Here's how the part is built. I have some questions about the finished solid (model axes, mm). Face numbers are marked on the shaded views. Round coordinates to 2 decimals unless told otherwise and drop trailing zeros. Write each loop counter-clockwise with the first axis right and the second up, starting at its lowest first coordinate (ties: lowest second). Pieces come first, ordered by that corner, then holes. Notation, with made-up numbers: (-13, -19) - (42, -19) arc R20 ccw to (42, 18) - close; hole circle Ø1 at (61.5, 25.5). An arc over 180 degrees is marked (long way). One line per item, written item: value. Start each with the question number.
Item 1: If I drill on line 1 (Z direction, x = -4, y = 10); line 2 (X direction, y = -0.5, z = 6); line 3 (Y direction, x = -14, z = 7.5), over which ranges is the centre line in solid material (lowest first)?
Item 2: Imagine slicing it at B-B, the plane x = 0. Please give me the cut outline in (y, z), then the cut area to 3 significant figures.
Item 3: For P1, Ø10, axis at x = 0.5, y = 0.5, coming from the +Z side, with a flat end and sliding along its axis, tell me the tip position at first contact or that it passes through.
Item 4: Thinking about a two-plate mould opening in X: for the marked faces 1, 2, 3 and 4, which applies, released by +X, released by -X, zero draft, split by the parting line, or undercut?
Item 5: Imagine slicing it at A-A, the plane z = 10.25. Please give me the cut outline in (x, y).
```python
from build123d import *

# Parameters (mm, degrees)
F0_W     = 74
F0_H     = 37
F1_DEPTH = 16
F2_T     = -1.5
F3_W     = 74
F3_H     = 37
F3_W_2   = 72
F3_H_2   = 35
F4_DEPTH = 2
F5_R     = 2


with BuildPart() as f1:
    # F0 (on Top) → F1 (new body)
    with BuildSketch(Plane.XY):
        Rectangle(F0_W, F0_H)
    extrude(amount=F1_DEPTH)

    # F2 (hollow: no face is removed)
    offset(amount=F2_T, mode=Mode.SUBTRACT)

    # F3 (on face) → F4 (join)
    with BuildSketch(Plane.XY.offset(16)):
        Rectangle(F3_W, F3_H)
        Rectangle(F3_W_2, F3_H_2, mode=Mode.SUBTRACT)
    extrude(amount=F4_DEPTH)

    # F5
    f5_edges = [f1.edges().sort_by_distance(p)[0] for p in [
        (-37, -18.5, 9),
        (36, 17.5, 17),
        (-36, 17.5, 17),
        (-36, -17.5, 17),
        (36, -17.5, 17),
        (37, -18.5, 9),
        (-37, 18.5, 9),
        (37, 18.5, 9),
    ]]
    fillet(f5_edges, radius=F5_R)


solid = f1.part
```
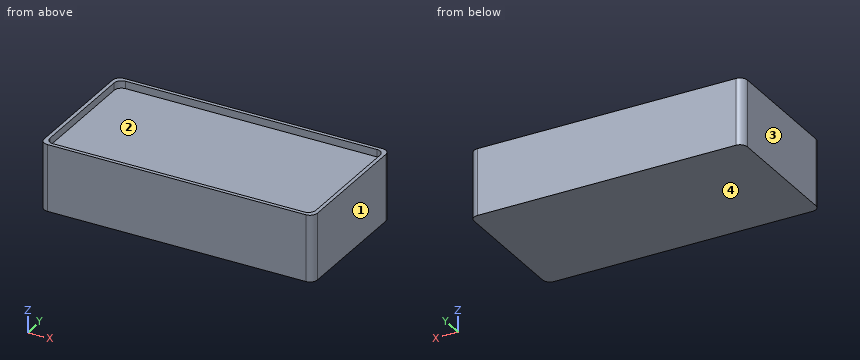
Values follow:
1. line 1: z = 0 to 1.5, 14.5 to 16
1. line 2: x = -37 to -35.5, 35.5 to 37
1. line 3: y = -18.5 to -17, 17 to 18.5
2. outline: (-18.5, 0) - (18.5, 0) - (18.5, 18) - (17.5, 18) - (17.5, 16) - (-17.5, 16) - (-17.5, 18) - (-18.5, 18) - close; hole (-17, 1.5) - (17, 1.5) - (17, 14.5) - (-17, 14.5) - close
2. area: 154 mm^2
3. P1: stops at z = 16
4. face 1: released by +X
4. face 2: undercut
4. face 3: released by -X
4. face 4: zero draft
5. outline: (-37, -16.5) arc R2 ccw to (-35, -18.5) - (35, -18.5) arc R2 ccw to (37, -16.5) - (37, 16.5) arc R2 ccw to (35, 18.5) - (-35, 18.5) arc R2 ccw to (-37, 16.5) - close; hole (-35.5, -17) - (35.5, -17) - (35.5, 17) - (-35.5, 17) - close
